Part model, mm, in its own coordinate system. Face numbers are marked on the shaded views. A direction names the side the tool comes from. Round coordinates to 2 decimals unless told otherwise and drop trailing zeros. Loops run counter-clockwise (first coordinate to the right, second up) from the corner with the lowest first, then second, coordinate; pieces in that order, holes last. Notation, with made-up numbers: (4, 31.5) - (11, 31.5) arc R23 cw to (11, 44.5) - close; hole circle Ø5 at (25, 39.25). An arc over 180 degrees is marked (long way). Write each question's results on one line, items separated by ' | '. Start each with the question number.
(1) Drill centre lines: L1, parallel to Y at x = -34, z = -35; L2, parallel to X at y = 34, z = -28.5; L3, parallel to Y at x = 4.5, z = 29. Where is each one in solid material? Low to high.
(2) Cut at C-C, the plane z = -35.5. List the corners of the cut face in (x, y), then the cut area to 3 significant figures.
(3) Cut at A-A, the plane y = 13. List the corners of the cut face in (x, z).
(4) Cut at D-D, the plane z = 32. List the corners of the cut face in (x, y).
(5) Mould opens along X. For the marked faces 1, 2 and 3 say: released by +X, released by -X, zero draft, split by the parting line, or undercut.
(6) Cut at B-B, the plane x = 13. List the corners of the cut face in (y, z), then the cut area to 3 significant figures.
(7) Flat gauge pins, fed straight in: P1, Ø3, axis at x = -6, y = 7.5, coming from the -Z side; P2, Ø3, axis at x = 27, z = 20.5, coming from the +Y side; P3, Ø4, axis at x = -10.5, z = 18, coming from the +Y side. Where does each tip first touch, or does it go through?
(8) Tool access for the marked faces 4 and 5: list every direction of +Z, -Z, +X, -X, +Y, -Y with a clear straight run to the whole face (end or side of a thin tool).
from build123d import *

# Parameters (mm, degrees)
ESBO_O1_W                = 70
ESBO_O1_H                = 90
RESSALTO_EXTRUS_O1_DEPTH = 55
CHANFRO1_SIZE            = 30
ESBO_O3_W                = 67
ESBO_O3_H                = 53.5
CORTE_EXTRUS_O1_DEPTH    = 58.5
ESBO_O5_W                = 67
ESBO_O5_H                = 22.5
CORTE_EXTRUS_O3_DEPTH    = 30
CHANFRO2_SIZE            = 31
ESBO_O4_R                = 8
CORTE_EXTRUS_O4_DEPTH    = 112.130553854
ESBO_O6_R                = 7.509542532
ESBO_O6_R_2              = 7.382654188
CORTE_EXTRUS_O5_DEPTH    = 100.749686716


with BuildPart() as part:
    # Esboço1 → Ressalto-extrusão1 (new body)
    with BuildSketch(Plane(origin=(0, 0, 0), x_dir=(1, 0, 0), z_dir=(0, 1, 0))):
        Rectangle(ESBO_O1_W, ESBO_O1_H)
    extrude(amount=RESSALTO_EXTRUS_O1_DEPTH)

    # Chanfro1
    chanfro1_edges = [part.edges().sort_by_distance(p)[0] for p in [
        (0, 55, 45),
    ]]
    chamfer(chanfro1_edges, length=CHANFRO1_SIZE)

    # Esboço3 → Corte-extrusão1 (cut)
    with BuildSketch(Plane(origin=(0, 0, -45), x_dir=(-1, 0, 0), z_dir=(0, 0, -1))):
        with Locations((0, 28.25)):
            Rectangle(ESBO_O3_W, ESBO_O3_H)
    extrude(amount=-CORTE_EXTRUS_O1_DEPTH, mode=Mode.SUBTRACT)

    # Esboço5 → Corte-extrusão3 (cut)
    with BuildSketch(Plane(origin=(0, 0, 13.5), x_dir=(-1, 0, 0), z_dir=(0, 0, -1))):
        with Locations((0, 12.75)):
            Rectangle(ESBO_O5_W, ESBO_O5_H)
    extrude(amount=-CORTE_EXTRUS_O3_DEPTH, mode=Mode.SUBTRACT)

    # Chanfro2
    # the kernel refuses this chamfer: 31 mm, written as the material it takes off along each edge
    with BuildSketch(Plane(origin=(-33.5, 24, 13.5), x_dir=(0, -0.027495876610586407, 0.9996219169112968), z_dir=(1, 0, 0))) as chanfro2_piece_1_section:
        Polygon((CHANFRO2_SIZE * 0.999621916911, -CHANFRO2_SIZE * 0.0274958766106), (-CHANFRO2_SIZE * 0.0274958766106, -CHANFRO2_SIZE * 0.999621916911), (0, 0), align=None)
    chanfro2_piece_1 = extrude(amount=67, mode=Mode.PRIVATE)
    chanfro2_piece_1 = split(chanfro2_piece_1, bisect_by=Plane(origin=(0, 34.34375, 43.5), z_dir=(0, 0, -1)), keep=Keep.TOP, mode=Mode.PRIVATE)
    add(chanfro2_piece_1, mode=Mode.SUBTRACT)

    # Esboço4 → Corte-extrusão4 (cut, through all)
    with BuildSketch(Plane.XY.offset(45)):
        with Locations((13, 13)):
            Circle(ESBO_O4_R)
        with Locations((-13, 13)):
            Circle(ESBO_O4_R)
    extrude(amount=-CORTE_EXTRUS_O4_DEPTH, mode=Mode.SUBTRACT)

    # Esboço6 → Corte-extrusão5 (cut, through all)
    with BuildSketch(Plane(origin=(35, 0, 0), x_dir=(0, 0, -1), z_dir=(1, 0, 0))):
        with Locations((35.5, 13)):
            Circle(ESBO_O6_R)
        with Locations((35.5, 39)):
            Circle(ESBO_O6_R_2)
    extrude(amount=-CORTE_EXTRUS_O5_DEPTH, mode=Mode.SUBTRACT)


solid = part.part
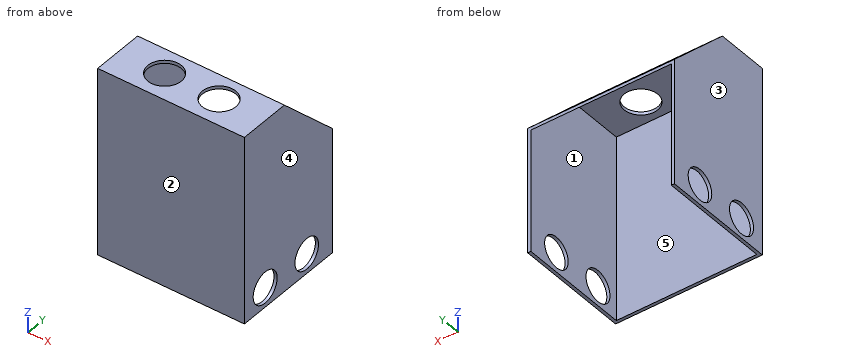
A:
1) L1: 0 to 5.51, 20.49 to 31.63, 46.37 to 55 | L2: -35 to -33.5, 33.5 to 35 | L3: 0 to 1.5, 39.5 to 41
2) outline: (-35, 0) - (35, 0) - (35, 5.49) - (33.5, 5.49) - (33.5, 1.5) - (-33.5, 1.5) - (-33.5, 5.49) - (-35, 5.49) - close; (-35, 20.51) - (-33.5, 20.51) - (-33.5, 31.62) - (-35, 31.62) - close; (-35, 46.38) - (-33.5, 46.38) - (-33.5, 55) - (-35, 55) - close; (33.5, 20.51) - (35, 20.51) - (35, 31.62) - (33.5, 31.62) - close; (33.5, 46.38) - (35, 46.38) - (35, 55) - (33.5, 55) - close | area: 176 mm2
3) outline: (-35, -45) - (-33.5, -45) - (-33.5, -43.01) - (-35, -43.01) - close; (-35, -27.99) - (-33.5, -27.99) - (-33.5, 43.5) - (-21, 43.5) - (-21, 45) - (-35, 45) - close; (-5, 43.5) - (5, 43.5) - (5, 45) - (-5, 45) - close; (21, 43.5) - (33.5, 43.5) - (33.5, -27.99) - (35, -27.99) - (35, 45) - (21, 45) - close; (33.5, -45) - (35, -45) - (35, -43.01) - (33.5, -43.01) - close
4) outline: (-35, 0) - (35, 0) - (35, 38) - (-35, 38) - close; hole (-33.5, 1.5) - (33.5, 1.5) - (33.5, 36.5) - (-33.5, 36.5) - close
5) face 1: undercut | face 2: zero draft | face 3: released by -X
6) outline: (0, -45) - (1.5, -45) - (1.5, 43.5) - (5, 43.5) - (5, 45) - (0, 45) - close; (21, 43.5) - (25, 43.5) - (55, 13.5) - (55, 15) - (25, 45) - (21, 45) - close | area: 191 mm2
7) P1: z = 43.5 | P2: y = 51 | P3: y = 54
8) face 4: +Z, -Z, +X, +Y, -Y | face 5: -Z
